Check sheet for the modelled part. Datum: model origin and axes. Units: mm. Round coordinates to 2 decimals unless told otherwise and drop trailing zeros. Order: outer loops, then holes, each group sorted by start corner. A loop starts at its lowest first (then second) coordinate and runs counter-clockwise, first axis right, second up. Notation, with made-up numbers: (30.25, -1) -> (82.25, -1) arc R16 cw to (82.25, 15) -> close; hole circle Ø10 at (38.5, -24.75). An arc over 180 degrees is marked (long way). Answer in a Markdown table with one row per item.
```python
from build123d import *

# Parameters (mm, degrees)
SKETCH_1_W          = 80
SKETCH_1_H          = 8
EXTRUDE_1_DEPTH     = 11.5
CUT_EXTRUDE_1_REACH = 83.217
SKETCH_2_R          = 1.55


with BuildPart() as part:
    # 草图1 → 凸台-拉伸1 (new body)
    with BuildSketch(Plane.XY):
        with Locations((40, 4)):
            Rectangle(SKETCH_1_W, SKETCH_1_H)
    extrude(amount=EXTRUDE_1_DEPTH)

    # 草图2 → 切除-拉伸1 (cut, up to next)
    with BuildSketch(Plane(origin=(0, 8, 0), x_dir=(1, 0, 0), z_dir=(0, 1, 0)), mode=Mode.PRIVATE) as cut_extrude_1_sk1:
        with Locations(Location((10, -5, 0), (0, 0, 270))):
            Circle(SKETCH_2_R)
    cut_extrude_1_tool1 = extrude(cut_extrude_1_sk1.sketch, amount=-CUT_EXTRUDE_1_REACH, mode=Mode.PRIVATE) & part.part
    # 草图2 → 切除-拉伸1 (cut, up to next)
    with BuildSketch(Plane(origin=(0, 8, 0), x_dir=(1, 0, 0), z_dir=(0, 1, 0)), mode=Mode.PRIVATE) as cut_extrude_1_sk2:
        with Locations(Location((70, -5, 0), (0, 0, 270))):
            Circle(SKETCH_2_R)
    cut_extrude_1_tool2 = extrude(cut_extrude_1_sk2.sketch, amount=-CUT_EXTRUDE_1_REACH, mode=Mode.PRIVATE) & part.part
    add(cut_extrude_1_tool1.solids().sort_by_distance((10, 8, 5))[0], mode=Mode.SUBTRACT)
    add(cut_extrude_1_tool2.solids().sort_by_distance((70, 8, 5))[0], mode=Mode.SUBTRACT)


solid = part.part
```
(1) Section check C-C on y = 2. Record the boundary of the cut face in (x, z).
Solutions:
| item | result |
|---|---|
| outline | (0, 0) -> (80, 0) -> (80, 11.5) -> (0, 11.5) -> close; hole circle Ø3.1 at (10, 5); hole circle Ø3.1 at (70, 5) |
(2) Depth check by flat-ended pin: pin 1 Ø6 at (x, z) = (39.5, 2) entering from -Y; pin 2 Ø1.9 at (x, z) = (10, 5) entering from +Y. Enter the tip coordinate at first touch or a pass-through.
Solutions:
| item | result |
|---|---|
| pin 1 | y = 0 |
| pin 2 | through |
(3) Scan lines: probe 1 along X at (y, z) = (2.5, 5); probe 2 along X at (y, z) = (7.75, 4); probe 3 along Z at (x, y) = (70, 5.5). Record each from-to range of solid material in increasing order. Write a range as from..to.
Solutions:
| item | result |
|---|---|
| probe 1 | 0..8.45, 11.55..68.45, 71.55..80 |
| probe 2 | 0..8.82, 11.18..68.82, 71.18..80 |
| probe 3 | 0..3.45, 6.55..11.5 |
(4) Section check B-B on z = 5.5. Record the boundary of the cut face in (x, y).
Solutions:
| item | result |
|---|---|
| outline | (0, 0) -> (8.53, 0) -> (8.53, 8) -> (0, 8) -> close; (11.47, 0) -> (68.53, 0) -> (68.53, 8) -> (11.47, 8) -> close; (71.47, 0) -> (80, 0) -> (80, 8) -> (71.47, 8) -> close |
(5) Section check A-A on x = 10. Record the boundary of the cut face in (y, z).
Solutions:
| item | result |
|---|---|
| outline | (0, 0) -> (8, 0) -> (8, 3.45) -> (0, 3.45) -> close; (0, 6.55) -> (8, 6.55) -> (8, 11.5) -> (0, 11.5) -> close |
(6) Draft check along Z on faces 1 (the cylindrical face through (71.537, 4.056, 4.798)), 2 (the flat face through (39, 4, 11.5)), 3 (the flat face through (39, 4, 0)). Enter one of: pulls with the +Z half, pulls with the -Z half, needs draft (parallel to the pull), parting line crosses it, or undercut.
Solutions:
| item | result |
|---|---|
| face 1 | undercut |
| face 2 | pulls with the +Z half |
| face 3 | pulls with the -Z half |
